Geometry: final body of the model. Coordinates: model frame, mm. Coordinates: 2 decimals unless noted, no trailing zeros. Loops run counter-clockwise (first coordinate to the right, second up) from the corner with the lowest first, then second, coordinate; pieces in that order, holes last. Notation, with made-up numbers: (7.5, 47) - (39.5, 47) arc R10 cw to (39.5, 54) - close; hole circle Ø6 at (20.25, -25.5). An arc over 180 degrees is marked (long way). Write each question's results on one line, items separated by ' | '. Start each with the question number.
from build123d import *

# Parameters (mm, degrees)
SKETCH1_R                                         = 57.15
BOSS_EXTRUDE1_DEPTH                               = 4.7625
CUT_EXTRUDE2_REACH                                = 82.963
CUT_EXTRUDE3_REACH                                = 82.661
CSK_FOR_4_FLAT_HEAD_MACHINE_SCREW_100_D           = 3.2639
CSK_FOR_4_FLAT_HEAD_MACHINE_SCREW_100_CSINK_D     = 5.715
CSK_FOR_4_FLAT_HEAD_MACHINE_SCREW_100_CSINK_ANGLE = 100


with BuildPart() as part:
    # Sketch1 → Boss-Extrude1 (new body)
    with BuildSketch(Plane(origin=(0, 0, 0), x_dir=(1, 0, 0), z_dir=(0, 1, 0))):
        with Locations(Location((0, 0, 0), (0, 0, 90))):
            Circle(SKETCH1_R)
    extrude(amount=BOSS_EXTRUDE1_DEPTH)

    # Sketch2 → Cut-Extrude2 (cut, up to next)
    with BuildSketch(Plane(origin=(0, 4.7625, 0), x_dir=(1, 0, 0), z_dir=(0, 1, 0)), mode=Mode.PRIVATE) as cut_extrude2_sk1:
        with BuildLine():
            Line((51.641532728, 6.985), (51.641532728, -6.985))
            Line((51.641532728, -6.985), (56.721532728, -6.985))
            ThreePointArc((56.721532728, -6.985), (57.15, 0), (56.721532728, 6.985))
            Line((56.721532728, 6.985), (51.641532728, 6.985))
        make_face()
    cut_extrude2_tool1 = extrude(cut_extrude2_sk1.sketch, amount=-CUT_EXTRUDE2_REACH, mode=Mode.PRIVATE) & part.part
    # Sketch2 → Cut-Extrude2 (cut, up to next)
    with BuildSketch(Plane(origin=(0, 4.7625, 0), x_dir=(1, 0, 0), z_dir=(0, 1, 0)), mode=Mode.PRIVATE) as cut_extrude2_sk2:
        with BuildLine():
            Line((-51.641532728, 6.985), (-56.721532728, 6.985))
            ThreePointArc((-56.721532728, 6.985), (-57.15, 0), (-56.721532728, -6.985))
            Line((-56.721532728, -6.985), (-51.641532728, -6.985))
            Line((-51.641532728, -6.985), (-51.641532728, 6.985))
        make_face()
    cut_extrude2_tool2 = extrude(cut_extrude2_sk2.sketch, amount=-CUT_EXTRUDE2_REACH, mode=Mode.PRIVATE) & part.part
    add(cut_extrude2_tool1.solids().sort_by_distance((54.325982, 4.7625, 0))[0], mode=Mode.SUBTRACT)
    add(cut_extrude2_tool2.solids().sort_by_distance((-54.325982, 4.7625, 0))[0], mode=Mode.SUBTRACT)

    # Sketch3 → Cut-Extrude3 (cut, up to next)
    with BuildSketch(Plane(origin=(0, 4.7625, 0), x_dir=(1, 0, 0), z_dir=(0, 1, 0)), mode=Mode.PRIVATE) as cut_extrude3_sk1:
        with BuildLine():
            Line((19.771578919, -48.215379233), (31.869953809, -41.230379233))
            Line((31.869953809, -41.230379233), (34.409953809, -45.629788284))
            ThreePointArc((34.409953809, -45.629788284), (28.575, -49.493351826), (22.311578919, -52.614788284))
            Line((22.311578919, -52.614788284), (19.771578919, -48.215379233))
        make_face()
    cut_extrude3_tool1 = extrude(cut_extrude3_sk1.sketch, amount=-CUT_EXTRUDE3_REACH, mode=Mode.PRIVATE) & part.part
    # Sketch3 → Cut-Extrude3 (cut, up to next)
    with BuildSketch(Plane(origin=(0, 4.7625, 0), x_dir=(1, 0, 0), z_dir=(0, 1, 0)), mode=Mode.PRIVATE) as cut_extrude3_sk2:
        with BuildLine():
            Line((-31.869953809, 41.230379233), (-34.409953809, 45.629788284))
            ThreePointArc((-34.409953809, 45.629788284), (-28.575, 49.493351826), (-22.311578919, 52.614788284))
            Line((-22.311578919, 52.614788284), (-19.771578919, 48.215379233))
            Line((-19.771578919, 48.215379233), (-31.869953809, 41.230379233))
        make_face()
    cut_extrude3_tool2 = extrude(cut_extrude3_sk2.sketch, amount=-CUT_EXTRUDE3_REACH, mode=Mode.PRIVATE) & part.part
    add(cut_extrude3_tool1.solids().sort_by_distance((27.162991, 4.7625, 47.04768))[0], mode=Mode.SUBTRACT)
    add(cut_extrude3_tool2.solids().sort_by_distance((-27.162991, 4.7625, -47.04768))[0], mode=Mode.SUBTRACT)

    # CSK for #4 Flat Head Machine Screw (100)1 (through all)
    with Locations(Plane(origin=(0, 4.7625, 0), x_dir=(1, 0, 0), z_dir=(0, 1, 0))):
        with Locations((25.4, 0), (0, -25.4), (0, 25.4), (-25.4, 0)):
            CounterSinkHole(CSK_FOR_4_FLAT_HEAD_MACHINE_SCREW_100_D / 2, CSK_FOR_4_FLAT_HEAD_MACHINE_SCREW_100_CSINK_D / 2, counter_sink_angle=CSK_FOR_4_FLAT_HEAD_MACHINE_SCREW_100_CSINK_ANGLE)


solid = part.part
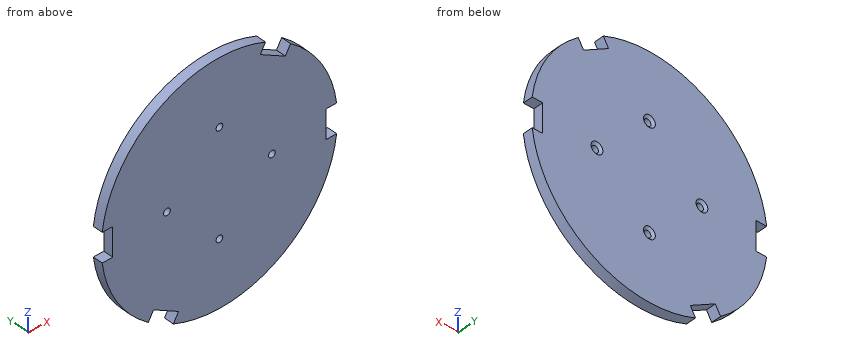
1) Material intervals for line 1 (Z direction, x = 0, y = 1.8); line 2 (X direction, y = 2.9, z = -25.4); line 3 (X direction, y = 0.7, z = 28.5), sorted ascending. Write a range as [from, to].
2) Pin query (flat end, axial travel): pin 1 Ø10 at (x, z) = (18, 40) entering from -Y; pin 2 Ø5 at (x, z) = (-25.4, 0) entering from +Y; pin 3 Ø1.5 at (x, y) = (4, 2) entering from -Z; pin 4 Ø4 at (x, z) = (0, 25.4) entering from +Y. Return the tip coordinate at first contact, or that it passes through.
3) Section query D-D on x = 25.4. Output: boundary loops of the cut face in (y, z), and give its area (3 significant figures).
4) Section query C-C on z = -25.4. Output: boundary loops of the cut face in (x, y), and give its area (3 significant figures).
5) Section query B-B on x = 0. Output: boundary loops of the cut face in (y, z), and give its area (3 significant figures).
6) Section query A-A on y = 1. Output: boundary loops of the cut face in (x, z) (3 decimals).
Returned:
1) line 1: z = [-57.15, -27.03], [-23.77, 23.77], [27.03, 57.15] | line 2: x = [-51.2, -1.63], [1.63, 51.2] | line 3: x = [-49.54, 49.54]
2) pin 1: stops at y = 0 | pin 2: stops at y = 4.46 | pin 3: stops at z = -57.06 | pin 4: stops at y = 4.04
3) outline: (0, -51.2) - (4.76, -51.2) - (4.76, -2.86) - (3.73, -1.63) - (0, -1.63) - close; (0, 1.63) - (3.73, 1.63) - (4.76, 2.86) - (4.76, 44.97) - (0, 44.97) - close | area: 441 mm²
4) outline: (-51.2, 0) - (-1.63, 0) - (-1.63, 3.73) - (-2.86, 4.76) - (-51.2, 4.76) - close; (1.63, 0) - (51.2, 0) - (51.2, 4.76) - (2.86, 4.76) - (1.63, 3.73) - close | area: 471 mm²
5) outline: (0, -57.15) - (4.76, -57.15) - (4.76, -28.26) - (3.73, -27.03) - (0, -27.03) - close; (0, -23.77) - (3.73, -23.77) - (4.76, -22.54) - (4.76, 22.54) - (3.73, 23.77) - (0, 23.77) - close; (0, 27.03) - (3.73, 27.03) - (4.76, 28.26) - (4.76, 57.15) - (0, 57.15) - close | area: 511 mm²
6) outline: (-56.722, -6.985) arc R57.15 ccw to (-34.41, -45.63) - (-31.87, -41.23) - (-19.772, -48.215) - (-22.312, -52.615) arc R57.15 ccw to (56.722, -6.985) - (51.642, -6.985) - (51.642, 6.985) - (56.722, 6.985) arc R57.15 ccw to (34.41, 45.63) - (31.87, 41.23) - (19.772, 48.215) - (22.312, 52.615) arc R57.15 ccw to (-56.722, 6.985) - (-51.642, 6.985) - (-51.642, -6.985) - close; hole circle Ø3.264 at (-25.4, 0); hole circle Ø3.264 at (0, -25.4); hole circle Ø3.264 at (0, 25.4); hole circle Ø3.264 at (25.4, 0)
